Model file for the job. Use its own axes, mm. Face numbers are marked on the shaded views. A direction names the side the tool comes from. Give positions to 0.01 mm unless a question says otherwise; leave off trailing zeros. Use CSV: the item, a comma, the result in double quotes. Start each with the question number.
1. Wall check: line 1 (X direction, y = -5.5, z = -1.9); line 2 (Z direction, x = 7.5, y = -9); line 3 (Y direction, x = 5.75, z = -2.1). Give the ranges that are in metal, low to high. Write a range as from..to.
2. Drop flat-ended pins along their axis: pin 1 (1.2 mm diameter, centred on y = 14.5, z = -1, fed in from -X); pin 2 (0.8 mm diameter, centred on x = 0.5, z = -0.5, fed in from -Y); pin 3 (1.1 mm diameter, centred on x = -1.5, z = -2, fed in from +Y). Give the stop position or say it passes through.
3. Pull direction X, two halves, no side cores. Call the marked faces 3 and 4: released by +X, released by -X, zero draft, split by the parting line, or undercut.
4. 3-axis set-ups, long thin cutter, end or side, ignore diameter. For the marked faces 1 and 2: which of +Z, -Z, +X, -X, +Y, -Y reach the whole face in a straight line?
```python
from build123d import *

# Parameters (mm, degrees)
F1_DEPTH = 1
F2_W     = 0.6565612018
F2_H     = 2.5395583361
F2_W_2   = 0.6960576609
F2_W_3   = 0.8317038625
F2_H_2   = 3.7825570011
F2_W_4   = 0.7836289912
F3_DEPTH = 2.5
F2_W_5   = 7
F2_H_3   = 1.2
F4_DEPTH = 2.6
F6_DEPTH = 1
F7_R     = 0.99999
F8_W     = 11
F8_H     = 6.2
F9_DEPTH = 6


# Not quite as in the source:
# - a fillet or chamfer is up to 0.001 mm smaller than in the source, because OpenCascade refuses the exact size


with BuildPart() as f1:
    # F0 (on Top) → F1 (new body)
    with BuildSketch(Plane.XY):
        with BuildLine():
            ThreePointArc((10.5534817095, 15.4336250836), (0, 24.3689653978), (-10.5534817095, 15.4336250836))
            Line((-10.5534817095, 15.4336250836), (-13.6603478203, -3.1468722986))
            ThreePointArc((-13.6603478203, -3.1468722986), (0, -19.2810346022), (13.6603478203, -3.1468722986))
            Line((13.6603478203, -3.1468722986), (10.5534817095, 15.4336250836))
        make_face()
        with BuildLine():
            ThreePointArc((-12.1808877675, -3.3942544975), (-10.7458713669, 0.6557337165), (-8.0101498113, 3.9689653978))
            ThreePointArc((-8.0101498113, 3.9689653978), (-7.3298242511, 6.556361809), (-8.0101498113, 9.1437582202))
            ThreePointArc((-8.0101498113, 9.1437582202), (-9.0606365073, 12.0737017575), (-9.0740216568, 15.1862428847))
            ThreePointArc((-9.0740216568, 15.1862428847), (0, 22.8689653978), (9.0740216568, 15.1862428847))
            ThreePointArc((9.0740216568, 15.1862428847), (9.0606535532, 12.0737985759), (8.0102465186, 9.1439294077))
            ThreePointArc((8.0102465186, 9.1439294077), (8.0101981654, 9.1438438137), (8.0101498113, 9.1437582202))
            ThreePointArc((8.0101498113, 9.1437582202), (7.3298242511, 6.556361809), (8.0101498113, 3.9689653978))
            ThreePointArc((8.0101498113, 3.9689653978), (10.7458713669, 0.6557337165), (12.1808877675, -3.3942544975))
            ThreePointArc((12.1808877675, -3.3942544975), (0, -17.7810346022), (-12.1808877675, -3.3942544975))
        make_face(mode=Mode.SUBTRACT)
        with BuildLine():
            Line((8.0101498113, 3.9689653978), (-8.0101498113, 3.9689653978))
            ThreePointArc((-8.0101498113, 3.9689653978), (-10.7458713669, 0.6557337165), (-12.1808877675, -3.3942544975))
            ThreePointArc((-12.1808877675, -3.3942544975), (0, -17.7810346022), (12.1808877675, -3.3942544975))
            ThreePointArc((12.1808877675, -3.3942544975), (10.7458713669, 0.6557337165), (8.0101498113, 3.9689653978))
        make_face()
        with BuildLine():
            ThreePointArc((-8.0101498113, 9.1437582202), (-7.3298242511, 6.556361809), (-8.0101498113, 3.9689653978))
            Line((-8.0101498113, 3.9689653978), (8.0101498113, 3.9689653978))
            ThreePointArc((8.0101498113, 3.9689653978), (7.3298242511, 6.556361809), (8.0101498113, 9.1437582202))
            ThreePointArc((8.0101498113, 9.1437582202), (0, 4.4689653978), (-8.0101498113, 9.1437582202))
        make_face()
        with BuildLine():
            ThreePointArc((-9.0740216568, 15.1862428847), (-9.0606365073, 12.0737017575), (-8.0101498113, 9.1437582202))
            ThreePointArc((-8.0101498113, 9.1437582202), (0, 4.4689653978), (8.0101498113, 9.1437582202))
            ThreePointArc((8.0101498113, 9.1437582202), (8.0101981654, 9.1438438137), (8.0102465186, 9.1439294077))
            ThreePointArc((8.0102465186, 9.1439294077), (9.0606535532, 12.0737985759), (9.0740216568, 15.1862428847))
            ThreePointArc((9.0740216568, 15.1862428847), (0, 22.8689653978), (-9.0740216568, 15.1862428847))
        make_face()
    extrude(amount=-F1_DEPTH)

    # F2 (on face) → F3 (join)
    with BuildSketch(Plane.XY):
        with BuildLine():
            ThreePointArc((-12.0822570973, -3.4107466441), (-11.6589837477, -9.190103366), (-8.626729972, -14.1282772682))
            ThreePointArc((-8.626729972, -14.1282772682), (-8.5678329378, -14.1863038014), (-8.5085456051, -14.2439314975))
            ThreePointArc((-8.5085456051, -14.2439314975), (-7.5199061996, -15.9719752427), (-5.65, -16.6553447357))
            Line((-5.65, -16.6553447357), (5.65, -16.6553447357))
            ThreePointArc((5.65, -16.6553447357), (7.5199061996, -15.9719752427), (8.5085456051, -14.2439314975))
            ThreePointArc((8.5085456051, -14.2439314975), (8.5678329378, -14.1863038014), (8.626729972, -14.1282772682))
            ThreePointArc((8.626729972, -14.1282772682), (11.6589837477, -9.190103366), (12.0822570973, -3.4107466441))
            Line((12.0822570973, -3.4107466441), (8.9753909866, 15.1697507381))
            ThreePointArc((8.9753909866, 15.1697507381), (0, 22.7689653978), (-8.9753909866, 15.1697507381))
            Line((-8.9753909866, 15.1697507381), (-12.0822570973, -3.4107466441))
        make_face()
        with Locations((-8.9782806009, -11.8910893798)):
            Rectangle(F2_W, F2_H, mode=Mode.SUBTRACT)
        with Locations((8.9980288304, -11.8910893798)):
            Rectangle(F2_W_2, F2_H, mode=Mode.SUBTRACT)
        with Locations((-9.0658519313, 9.3533767637)):
            Rectangle(F2_W_3, F2_H_2, mode=Mode.SUBTRACT)
        with Locations((9.0418144956, 9.3533767637)):
            Rectangle(F2_W_4, F2_H_2, mode=Mode.SUBTRACT)
        with Locations((-9.0658519313, 9.3533767637)):
            Rectangle(F2_W_3, F2_H_2)
        with Locations((9.0418144956, 9.3533767637)):
            Rectangle(F2_W_4, F2_H_2)
        with Locations((8.9980288304, -11.8910893798)):
            Rectangle(F2_W_2, F2_H)
        with Locations((-8.9782806009, -11.8910893798)):
            Rectangle(F2_W, F2_H)
    extrude(amount=-F3_DEPTH)

    # F2 (on face) → F4 (join)
    with BuildSketch(Plane.XY):
        with BuildLine():
            Line((3.5, -17.9553447357), (-3.5, -17.9553447357))
            Line((-3.5, -17.9553447357), (-3.5, -18.831501012))
            ThreePointArc((-3.5, -18.831501012), (0, -19.2810346022), (3.5, -18.831501012))
            Line((3.5, -18.831501012), (3.5, -17.9553447357))
        make_face()
        with Locations((0, -17.3553447357)):
            Rectangle(F2_W_5, F2_H_3)
    extrude(amount=-F4_DEPTH)

    # F5 (on face) → F6 (cut)
    with BuildSketch(Plane(origin=(0, 0, -2.5), x_dir=(1, 0, 0), z_dir=(0, 0, -1))):
        with BuildLine():
            Line((-10.602797021, 3.658128847), (-7.4959309103, -14.9223685352))
            ThreePointArc((-7.4959309103, -14.9223685352), (0, -21.2689653739), (7.4959309103, -14.9223685352))
            Line((7.4959309103, -14.9223685352), (10.602797021, 3.658128847))
            ThreePointArc((10.602797021, 3.658128847), (10.1137042336, 9.0745886584), (7.0360940107, 13.5585114899))
            ThreePointArc((7.0360940107, 13.5585114899), (6.7072526833, 14.6730683852), (5.65, 15.1553447118))
            Line((5.65, 15.1553447118), (-5.65, 15.1553447118))
            ThreePointArc((-5.65, 15.1553447118), (-6.7072526833, 14.6730683852), (-7.0360940107, 13.5585114899))
            ThreePointArc((-7.0360940107, 13.5585114899), (-10.1137042336, 9.0745886584), (-10.602797021, 3.658128847))
        make_face()
    extrude(amount=-F6_DEPTH, mode=Mode.SUBTRACT)

    # F7 (radius 1 in the source; OpenCascade refuses exactly that, so slightly less here)
    f7_edges = [f1.edges().sort_by_distance(p)[0] for p in [
        (0, -19.281035, 0),
        (0, 24.368965, 0),
        (12.106915, 6.143376, 0),
        (-12.106915, 6.143376, 0),
    ]]
    fillet(f7_edges, radius=F7_R)

    # F8 (on face) → F9 (cut)
    with BuildSketch(Plane.XY):
        with Locations((0, 15.7622105017)):
            Rectangle(F8_W, F8_H)
    extrude(amount=-F9_DEPTH, mode=Mode.SUBTRACT)


solid = f1.part
```
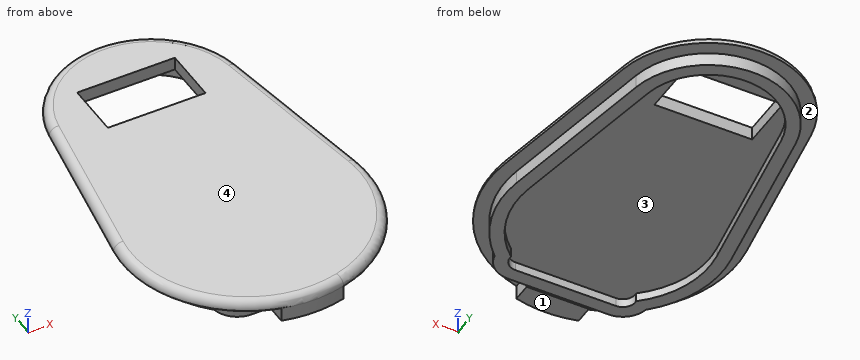
Verdict:
1,line 1,"-12.25..-10.75, 10.75..12.25"
1,line 2,"-1.5..0"
1,line 3,"-16.65..-15.15, 18.64..20.72"
2,pin 1,"x = -10.81"
2,pin 2,"y = -19.27"
2,pin 3,"y = 22.72"
3,face 3,"undercut"
3,face 4,"zero draft"
4,face 1,"-Z, +X, -X, +Y, -Y"
4,face 2,"-Z"
